Autodesk Inventor part; units mm, degrees
ref_plane "Work Plane1" through (127.45, 59.5, 9.9) normal (0, 1, 0) x (1, 0, 0)
ref_plane "YZ Plane" through (0, 0, 0) normal (1, 0, 0) x (0, 1, 0)
ref_plane "XZ Plane" through (0, 0, 0) normal (0, 1, 0) x (-1, 0, 0)
sketch "Sketch1" plane through (0, 0, 0) normal (0, 1, 0) x (-1, 0, 0)
  line L0 (-113.9895, -20.65) -> (-113.9895, -0.1)
  line L1 (-105.9, -20.65) -> (-113.9895, -20.65)
  line L2 (-105.9, -20.65) -> (-105.9, -19.5)
  line L3 (-105.9, -19.5) -> (-112.525, -19.5)
  line L4 (-112.525, -19.5) -> (-112.525, 19.5)
  line L5 (-112.525, 19.5) -> (-73.775, 19.5)
  line L6 (-127.45, 19.9) -> (-115.3, 19.9)
  line L7 (-115.3, 19.9) -> (-115.3, 9.9)
  line L8 (-115.3, 9.9) -> (-127.45, 9.9)
  line L9 (-127.45, 9.9) -> (-127.45, 19.9)
  line L10 (-124.5373, 9.9) -> (-126.375, 9.9)
  arc A0 (-124.8248, 9.9909) -> (-124.5373, 9.9) centre (-124.5373, 10.4) ccw
  arc A1 (-127.375, 14.9) -> (-124.8248, 9.9909) centre (-121.375, 14.9) ccw
  line L11 (-127.375, 10.9) -> (-127.375, 14.9)
  arc A2 (-127.375, 10.9) -> (-126.375, 9.9) centre (-126.375, 10.9) ccw
  line L12 (-127.375, 14.9) -> (-127.375, 18.9)
  arc A3 (-124.8248, 19.8091) -> (-127.375, 14.9) centre (-121.375, 14.9) ccw
  arc A4 (-124.5373, 19.9) -> (-124.8248, 19.8091) centre (-124.5373, 19.4) ccw
  line L13 (-126.375, 19.9) -> (-124.5373, 19.9)
  arc A5 (-126.375, 19.9) -> (-127.375, 18.9) centre (-126.375, 18.9) ccw
  line L14 (-118.2127, 19.9) -> (-116.375, 19.9)
  arc A6 (-117.9252, 19.8091) -> (-118.2127, 19.9) centre (-118.2127, 19.4) ccw
  arc A7 (-115.375, 14.9) -> (-117.9252, 19.8091) centre (-121.375, 14.9) ccw
  line L15 (-115.375, 18.9) -> (-115.375, 14.9)
  arc A8 (-115.375, 18.9) -> (-116.375, 19.9) centre (-116.375, 18.9) ccw
  line L16 (-115.375, 14.9) -> (-115.375, 10.9)
  arc A9 (-117.9252, 9.9909) -> (-115.375, 14.9) centre (-121.375, 14.9) ccw
  arc A10 (-118.2127, 9.9) -> (-117.9252, 9.9909) centre (-118.2127, 10.4) ccw
  line L17 (-116.375, 9.9) -> (-118.2127, 9.9)
  arc A11 (-116.375, 9.9) -> (-115.375, 10.9) centre (-116.375, 10.9) ccw
  arc A12 (-118.2127, 9.9) -> (-117.9252, 9.9909) centre (-118.2127, 10.4) ccw
  arc A13 (-117.9252, 9.9909) -> (-117.9252, 19.8091) centre (-121.375, 14.9) ccw
  arc A14 (-117.9252, 19.8091) -> (-118.2127, 19.9) centre (-118.2127, 19.4) ccw
  line L18 (-118.2127, 19.9) -> (-124.5373, 19.9)
  arc A15 (-124.5373, 19.9) -> (-124.8248, 19.8091) centre (-124.5373, 19.4) ccw
  arc A16 (-124.8248, 19.8091) -> (-124.8248, 9.9909) centre (-121.375, 14.9) ccw
  arc A17 (-124.8248, 9.9909) -> (-124.5373, 9.9) centre (-124.5373, 10.4) ccw
  line L19 (-124.5373, 9.9) -> (-118.2127, 9.9)
  line L20 (-73.775, 19.5) -> (-73.775, 20.65)
  line L21 (-115.3, 19.9) -> (-115.3, 9.9)
  line L22 (-115.3, 9.9) -> (-114.3, 9.9)
  line L23 (-114.3, 9.9) -> (-114.3, 19.9)
  line L24 (-114.3, 19.9) -> (-115.3, 19.9)
  line L25 (-121.375, 14.9) -> (-121.375, 19.9)
  arc A18 (-114.3, 16.3047) -> (-115.6679, 19.6071) centre (-118.9703, 16.3047) ccw
  arc A19 (-116.375, 19.9) -> (-117.9252, 19.8091) centre (-116.375, 6.6367) ccw
  line L26 (-127.45, 19.9) -> (-127.45, 9.9)
  line L27 (-127.45, 9.9) -> (-128.45, 9.9)
  line L28 (-128.45, 9.9) -> (-128.45, 19.9)
  line L29 (-128.45, 19.9) -> (-127.45, 19.9)
  arc A20 (-127.0821, 19.6071) -> (-128.45, 16.3047) centre (-123.7797, 16.3047) ccw
  arc A21 (-124.8248, 19.8091) -> (-126.375, 19.9) centre (-126.375, 6.6367) ccw
  line L30 (-114.3, 9.9) -> (-128.45, 9.9)
  line L31 (-128.45, 9.9) -> (-128.45, -0.1)
  line L32 (-128.45, -0.1) -> (-114.3, -0.1)
  line L33 (-114.3, -0.1) -> (-114.3, 9.9)
  line L34 (-121.375, 9.9) -> (-121.375, -0.1)
  circle A22 centre (-121.375, 4.9) radius 1.5
  circle A23 centre (-121.375, 4.9) radius 3
  arc A24 (-121.375, -0.1) -> (-114.3, 6.975) centre (-121.375, 6.975) ccw
  arc A25 (-128.45, 6.975) -> (-121.375, -0.1) centre (-121.375, 6.975) ccw
  line L35 (-128.9145, -0.1) -> (-128.9145, 20.65)
  line L36 (-128.9145, -0.1) -> (-113.9895, -0.1)
  line L37 (-128.9145, 20.65) -> (-73.775, 20.65)
  circle A26 centre (-121.375, 4.9163) radius 1.4375
  point P0 (0, 0)
  point P1 (-135.6645, 14.9)
  dimension "d18" = 1
  dimension "d20" = 3
  dimension "d21" = 6
  dimension "d22" = 10
ref_plane "Work Plane1" through (127.45, 59.5, 9.9) normal (0, 1, 0) x (1, 0, 0)
extrude "Extrusion1" add sketch "Sketch1" along normal blind 6 from surface at 59.5 contours A25 L31 L27 L8 L34 A23 | L34 A23 L8 L22 L33 A24 | A23 L34 A22 | L34 A22 A23 | L22 L7 A18 L23 | L28 A20 L9 L27 | L8 A11 L16 L15 A8 A18 L7 | L9 A20 A5 L12 L11 A2 L8 | L8 A10 A9 L16 A11 | L8 A2 L11 A1 A0 | A8 L15 A7 A19 | A5 A21 A3 L12
fillet "Fillet1" radius 0.5 2 edges at (117.9252, 62.5, 19.8091) (124.8248, 62.5, 19.8091)
sketch "Sketch2" plane through (118.1857, 65.5, 20.6175) normal (0, 1, 0) x (1, 0, 0)
  arc A0 (-0.2604, 10.6266) -> (-1.1435, 1.567) centre (3.1893, 5.7175) ccw
  arc A1 (0.0271, 10.7175) -> (-0.2604, 10.6266) centre (0.0271, 10.2175) ccw
  line L0 (6.3516, 10.7175) -> (0.0271, 10.7175)
  arc A2 (6.6391, 10.6266) -> (6.3516, 10.7175) centre (6.3516, 10.2175) ccw
  arc A3 (7.5222, 1.567) -> (6.6391, 10.6266) centre (3.1893, 5.7175) ccw
  circle A4 centre (3.1893, 15.7175) radius 3
  arc A5 (10.2643, 13.6425) -> (-3.8857, 13.6425) centre (3.1893, 13.6425) ccw
  line L1 (-3.8857, 4.3128) -> (-3.8857, 13.6425)
  arc A6 (-3.8857, 4.3128) -> (-2.5178, 1.0104) centre (0.7846, 4.3128) ccw
  arc A7 (-2.5178, 1.0104) -> (-1.8107, 0.7175) centre (-1.8107, 1.7175) ccw
  arc A8 (-1.8107, 0.7175) -> (-1.4926, 0.7213) centre (-1.8107, 13.9808) ccw
  arc A9 (7.8713, 0.7213) -> (8.1893, 0.7175) centre (8.1893, 13.9808) ccw
  arc A10 (8.1893, 0.7175) -> (8.8964, 1.0104) centre (8.1893, 1.7175) ccw
  arc A11 (8.8964, 1.0104) -> (10.2643, 4.3128) centre (5.5941, 4.3128) ccw
  line L2 (10.2643, 13.6425) -> (10.2643, 4.3128)
  line L3 (3.1893, 10.7175) -> (3.1893, 20.7175)
  arc A12 (7.5222, 1.567) -> (7.8713, 0.7213) centre (7.8833, 1.2212) ccw
  arc A13 (-1.4926, 0.7213) -> (-1.1435, 1.567) centre (-1.5046, 1.2212) ccw
  point P0 (-118.1857, 20.6175)
  dimension "d10" = 6
extrude "Extrusion2" add sketch "Sketch2" along normal blind 2 contours A0 A13 A8 A7 A6 L1 A5 L3 A4 L0 A1 | L3 A4 A5 L2 A11 A10 A9 A12 A3 A2 L0
properties part number "Z Stage Motor Clamp V5"
Design review of the part built by this model. Coordinates are the model's own, in mm. A direction names the side the tool comes from. Round coordinates to 2 decimals unless told otherwise and drop trailing zeros. Order: outer loops, then holes, each group sorted by start corner. A loop starts at its lowest first (then second) coordinate and runs counter-clockwise, first axis right, second up. Notation, with made-up numbers: (53.25, 75) - (71.25, 75) arc R23 cw to (71.25, 89) - close; hole circle Ø6 at (-27.5, 83). An arc over 180 degrees is marked (long way). Return JSON: item names as keys, results as strings.
Q1. The part is to be moulded in two halves that separate along Z. For faces 6 (the cylindrical face through (114.665, 63.444, 18.116)), 7 (the flat face through (120, 67.5, 8)), 8 (the cylindrical face through (126.955, 62.458, 17.107)), say which applies: pulls with the +Z half, pulls with the -Z half, needs draft (parallel to the pull), parting line crosses it, or undercut.
Computed values:
{"face 6": "pulls with the +Z half", "face 7": "needs draft", "face 8": "undercut"}
Q2. Machinability: for faces 1 (the flat face through (121, 59.5, 8)), 2 (the flat face through (121, 63, 9.9)), 3 (the flat face through (128.45, 63, 12)), 4 (the flat face through (123, 65.5, 4)), 5 (the cylindrical face through (125.61, 66.49, 19.59)), which of the approach directions +Z, -Z, +X, -X, +Y, -Y give a long, thin tool a straight path to every point of the face, cutting with its end or side? Answer none if there is none.
Computed values:
{"face 1": "+Z, -Z, +X, -X, -Y", "face 2": "+Z, +Y, -Y", "face 3": "+Z, -Z, +X, +Y, -Y", "face 4": "+Y", "face 5": "+Y, -Y"}
Q3. Consider section A-A on z = 16. Write out the cut boundary in (x, y), plus the area to 3 significant figures.
Computed values:
{"outline": "(114.3, 59.5) - (115.48, 59.5) - (115.48, 67.5) - (114.3, 67.5) - close; (127.27, 59.5) - (128.45, 59.5) - (128.45, 67.5) - (127.27, 67.5) - close", "area": "18.8 mm2"}
Q4. Wall thickness on L1, parallel to X at y = 62, z = 4.9 (3 decimals); L2, parallel to X at y = 62.5, z = 12; L3, parallel to Z at x = 116, y = 65.75: over which ranges is each line inside the solid? List them lowest first. Write a range as [from, to].
Computed values:
{"L1": "x = [114.611, 119.875], [122.875, 128.139]", "L2": "x = [114.3, 116.12], [126.63, 128.45]", "L3": "z = [2.37, 12.23], [17.57, 19.83]"}
Q5. For pin 1 Ø1.5 at (x, y) = (125.5, 60.5) entering from +Z; pin 2 Ø1.9 at (x, y) = (122.5, 63.5) entering from +Z, all flat-tipped, find the tip position at first contact; note any pin that passes through.
Computed values:
{"pin 1": "stops at z = 19.9", "pin 2": "stops at z = 9.9"}
Q6. Consider section B-B on x = 121.5. Write out the cut boundary in (y, z).
Computed values:
{"outline": "(59.5, -0.1) - (67.5, -0.1) - (67.5, 1.9) - (65.5, 1.9) - (65.5, 3.41) - (59.5, 3.41) - close; (59.5, 6.39) - (65.5, 6.39) - (65.5, 7.9) - (67.5, 7.9) - (67.5, 9.9) - (59.5, 9.9) - close"}
Q7. Consider section D-D on z = 12.75. Write out the cut boundary in (x, y), plus the area to 3 significant figures.
Computed values:
{"outline": "(114.3, 59.5) - (115.77, 59.5) - (115.77, 67.5) - (114.3, 67.5) - close; (126.98, 59.5) - (128.45, 59.5) - (128.45, 67.5) - (126.98, 67.5) - close", "area": "23.6 mm2"}
Q8. Consider section C-C on x = 119. Write out the cut boundary in (y, z).
Computed values:
{"outline": "(59.5, 0.31) - (67.5, 0.31) - (67.5, 3.07) - (65.5, 3.07) - (65.5, 6.73) - (67.5, 6.73) - (67.5, 9.9) - (59.5, 9.9) - close"}
